Here's how the part is built. I have some questions about the finished solid (model axes, mm). A direction names the side the tool comes from. Round coordinates to 2 decimals unless told otherwise and drop trailing zeros. Order: outer loops, then holes, each group sorted by start corner. A loop starts at its lowest first (then second) coordinate and runs counter-clockwise, first axis right, second up. Notation, with made-up numbers: (37, -9) - (74, -9) arc R20 ccw to (74, -3) - close; hole circle Ø5 at (13, 74.25). An arc over 180 degrees is marked (long way). Answer as a JSON object with one key per item and string values.
```python
from build123d import *

# Parameters (mm, degrees)
SKETCH_1_R      = 1.6
EXTRUDE_1_DEPTH = 10


with BuildPart() as part:
    # 草图1 → 凸台-拉伸1 (new body)
    with BuildSketch(Plane(origin=(0, 0, 0), x_dir=(0, 0, -1), z_dir=(1, 0, 0))):
        Polygon((-11.648969443, -15.638868598), (-18.351030557, -15.638868598), (-18.351030557, -4), (-32.84837567, -4), (-32.84837567, 9.413253291), (-59.646723814, 36.211601436), (-49.248051864, 46.610273387), (-14.086489785, 11.448711308), (6.718740299, 11.448711308), (29.902965659, 27.489458326), (42.078824949, 9.89128379), (22.001290309, -4), (18.351030557, -4), (18.351030557, -15.638868598), (11.648969443, -15.638868598), (11.648969443, -4), (-11.648969443, -4), align=None)
        with Locations((-15, -12)):
            Circle(SKETCH_1_R, mode=Mode.SUBTRACT)
        with Locations(Location((15, -12, 0), (0, 0, 180))):
            Circle(SKETCH_1_R, mode=Mode.SUBTRACT)
        with Locations((-48.060514381, 36.211601436)):
            Circle(SKETCH_1_R, mode=Mode.SUBTRACT)
        with Locations((-36.002441477, 25.143249656)):
            Circle(SKETCH_1_R, mode=Mode.SUBTRACT)
        with Locations((16.249207774, 5.411857631)):
            Circle(SKETCH_1_R, mode=Mode.SUBTRACT)
        with Locations((27.931653437, 14.600109184)):
            Circle(SKETCH_1_R, mode=Mode.SUBTRACT)
    extrude(amount=EXTRUDE_1_DEPTH)


solid = part.part
```
1. For P1, Ø6, axis at x = 8, y = 39, coming from the +Z side; P2, Ø6, axis at x = 4, y = 23.5, coming from the -Z side; P3, Ø1, axis at x = 8, y = 19, coming from the +Z side; P4, Ø1.9, axis at y = -12, z = 15, coming from the -X side, each with a flat end and sliding along its axis, tell me the tip position at first contact or that it passes through.
Responses:
{"P1": "z = 59.65", "P2": "z = -34.74", "P3": "z = 42.94", "P4": "through"}
2. For faces 1 (the face through (4.93, 29.276, 31.913)), 2 (the face through (5, -10, -18.351)), 3 (the face through (5, 3, 32.848)), which set-ups out of +Z, -Z, +X, -X, +Y, -Y let a thin tool reach every point of the face, with its end or its side?
Responses:
{"face 1": "+X, -X, +Y", "face 2": "-Z, +X, -X, -Y", "face 3": "+Z, +X, -X, -Y"}
3. Imagine slicing it at A-A (y = -12). List the corners of the cut face in (x, z) for me, plus the area to 3 significant figures.
Responses:
{"outline": "(0, -18.35) - (10, -18.35) - (10, -16.6) - (0, -16.6) - close; (0, -13.4) - (10, -13.4) - (10, -11.65) - (0, -11.65) - close; (0, 11.65) - (10, 11.65) - (10, 13.4) - (0, 13.4) - close; (0, 16.6) - (10, 16.6) - (10, 18.35) - (0, 18.35) - close", "area": "70.0 mm2"}
4. Imagine slicing it at C-C (z = -19.5). List the corners of the cut face in (x, y) for me.
Responses:
{"outline": "(0, -4) - (10, -4) - (10, 20.29) - (0, 20.29) - close"}
5. If I drill on L1, parallel to Y at x = 7.25, z = -15; L2, parallel to Z at x = 5.5, y = 36; L3, parallel to Z at x = 8.5, y = -11, over which ranges is the centre line in solid material (lowest first)? Write a range as [from, to].
Responses:
{"L1": "[-15.64, -13.6], [-10.4, 4.41], [6.41, 17.18]", "L2": "[38.64, 46.47], [49.65, 59.44]", "L3": "[-18.35, -16.25], [-13.75, -11.65], [11.65, 13.75], [16.25, 18.35]"}
6. Imagine slicing it at B-B (x = 6). List the corners of the cut face in (y, z) for me, plus the area to 3 significant figures.
Responses:
{"outline": "(-15.64, -18.35) - (-4, -18.35) - (-4, -22) - (9.89, -42.08) - (27.49, -29.9) - (11.45, -6.72) - (11.45, 14.09) - (46.61, 49.25) - (36.21, 59.65) - (9.41, 32.85) - (-4, 32.85) - (-4, 18.35) - (-15.64, 18.35) - (-15.64, 11.65) - (-4, 11.65) - (-4, -11.65) - (-15.64, -11.65) - close; hole circle Ø3.2 at (-12, -15); hole circle Ø3.2 at (-12, 15); hole circle Ø3.2 at (5.41, -16.25); hole circle Ø3.2 at (14.6, -27.93); hole circle Ø3.2 at (25.14, 36); hole circle Ø3.2 at (36.21, 48.06)", "area": "2,030 mm2"}
7. Imagine slicing it at D-D (y = 40). List the corners of the cut face in (x, z) for me, plus the area to 3 significant figures.
Responses:
{"outline": "(0, 42.64) - (10, 42.64) - (10, 55.86) - (0, 55.86) - close", "area": "132 mm2"}
8. Thinking about a two-plate mould opening in Y: for faces 4 (the face through (4.93, 18.81, -35.91)), 5 (the face through (10, 11, 9)), 6 (the face through (4.93, 37.56, 47.2)), 7 (the face through (5, -4, 0)), which applies, pulls with the +Y half, pulls with the -Y half, needs draft (parallel to the pull), parting line crosses it, or undercut?
Responses:
{"face 4": "pulls with the +Y half", "face 5": "needs draft", "face 6": "undercut", "face 7": "pulls with the -Y half"}
